from build123d import *

# Parameters (mm, degrees)
F1_DEPTH      = 10
F2_W          = 2
F2_H          = 10
F3_DEPTH      = 13.3
F3_DEPTH_BACK = 11.9
F4_R          = 4.99999


# Not quite as in the source:
# - a fillet or chamfer is up to 0.001 mm smaller than in the source, because OpenCascade refuses the exact size


with BuildPart() as f1:
    # F0 (on Top) → F1 (new body)
    with BuildSketch(Plane.XY):
        with BuildLine():
            Line((-1.25, -5.5), (3.25, -5.5))
            Line((3.25, -5.5), (3.25, 3.499999999))
            ThreePointArc((3.25, 3.499999999), (2.2500000005, 4.499999999), (1.25, 3.5))
            Line((1.25, 3.5), (1.25, -2.5))
            ThreePointArc((1.25, -2.5), (0.9571067812, -3.2071067812), (0.25, -3.5))
            Line((0.25, -3.5), (-0.25, -3.5))
            ThreePointArc((-0.25, -3.5), (-0.9571067812, -3.2071067812), (-1.25, -2.5))
            Line((-1.25, -2.5), (-1.25, 2.5))
            ThreePointArc((-1.25, 2.5), (-0.9571067812, 3.2071067812), (-0.25, 3.5))
            add(Edge.make_bspline(
                [(-1.2744928417, 5.5), (0.3231141309, 5.4264482222), (0.6423479063, 3.9560622536), (-0.25, 3.5)],
                knots=[0, 0, 0, 0, 2.2471282969, 2.2471282969, 2.2471282969, 2.2471282969], degree=3))
            ThreePointArc((-1.2744928417, 5.5), (-2.6728467387, 4.9056773399), (-3.25, 3.5001499804))
            Line((-3.25, 3.5001499804), (-3.25, -3.5))
            ThreePointArc((-3.25, -3.5), (-2.6642135624, -4.9142135624), (-1.25, -5.5))
        make_face()
    extrude(amount=F1_DEPTH)

    # F2 (on Front) → F3 (join, two sides)
    with BuildSketch(Plane.XZ) as f3_sk:
        with Locations((2.25, 5)):
            Rectangle(F2_W, F2_H)
    extrude(amount=F3_DEPTH)
    extrude(f3_sk.sketch, amount=-F3_DEPTH_BACK)

    # F4 (radius 5 in the source; OpenCascade refuses exactly that, so slightly less here)
    f4_edges = [f1.edges().sort_by_distance(p)[0] for p in [
        (2.25, -13.3, 10),
        (2.25, 11.9, 10),
        (2.25, -13.3, 0),
        (2.25, 11.9, 0),
    ]]
    fillet(f4_edges, radius=F4_R)


solid = f1.part
Read the model definition and answer for the solid it produces. Units are mm, in the model's axes. A direction names the side the tool comes from. Coordinates: 2 decimals unless noted, no trailing zeros. Loops run counter-clockwise (first coordinate to the right, second up) from the corner with the lowest first, then second, coordinate; pieces in that order, holes last. Notation, with made-up numbers: (-16.5, 78.5) - (11.5, 78.5) arc R30 ccw to (11.5, 111.5) - close; hole circle Ø3 at (44.25, 73). An arc over 180 degrees is marked (long way). Answer in a Markdown table with one row per item.
Q1. For faces 4 (the flat face through (2, -1, 0)), 5 (the flat face through (0, -5.5, 5)), 6 (the cylindrical face through (-0.949, -3.215, 4.93)), 7 (the flat face through (1.25, 5, 5)), 8 (the cylindrical face through (2.26, -11.8, 8.57)), determine the directions among +Z, -Z, +X, -X, +Y, -Y from which every point of the face is accessible in a straight line to the end or side of a thin tool.
Here are the results:
| item | result |
|---|---|
| face 4 | -Z, +X, -X, +Y, -Y |
| face 5 | +Z, -Z, -X, -Y |
| face 6 | +Z, -Z |
| face 7 | +Z, -Z, +Y |
| face 8 | +Z, +X, -X, -Y |
Q2. Find section C-C on y = -7.5. Write down the section's boundary in (x, z).
Here are the results:
| item | result |
|---|---|
| outline | (1.25, 0) - (3.25, 0) - (3.25, 10) - (1.25, 10) - close |
Q3. Find section D-D on x = -2.5. Write down the section's boundary in (y, z), plus the area to 3 significant figures.
Here are the results:
| item | result |
|---|---|
| outline | (-5.06, 0) - (5.06, 0) - (5.06, 10) - (-5.06, 10) - close |
| area | 101 mm^2 |
Q4. Find section A-A on y = -1. Write down the section's boundary in (x, z).
Here are the results:
| item | result |
|---|---|
| outline | (-3.25, 0) - (-1.25, 0) - (-1.25, 10) - (-3.25, 10) - close; (1.25, 0) - (3.25, 0) - (3.25, 10) - (1.25, 10) - close |
Q5. The mould has two halves that part along X. Classify faces 1 (the flat face through (3.25, -1, 5)), 2 (the cylindrical face through (-0.965, 3.199, 4.93)), 3 (the flat face through (1.25, -9, 5)): pulls with the +X half, pulls with the -X half, needs draft (parallel to the pull), parting line crosses it, or undercut.
Here are the results:
| item | result |
|---|---|
| face 1 | pulls with the +X half |
| face 2 | undercut |
| face 3 | pulls with the -X half |
Q6. Given P1, Ø2.5, axis at y = -11, z = 3.5, coming from the -X side; P2, Ø3, axis at x = -0.5, z = 2, coming from the +Y side; P3, Ø1.2, axis at x = -0.5, z = 3, coming from the -Y side, each flat-ended and moving along its own axis, determine where each tip first touches the part or whether it passes through.
Here are the results:
| item | result |
|---|---|
| P1 | stops at x = 1.25 |
| P2 | stops at y = 5.5 |
| P3 | stops at y = -5.5 |
Q7. Straight lines are drawn through the part: line 1 along X through (y, z) = (2.5, 3); line 2 along X through (y, z) = (-11.25, 6.25); line 3 along Y through (x, z) = (-0.75, 5.25). For each, find the intervals that lie inside material, in ascending order. Write a range as [from, to].
Here are the results:
| item | result |
|---|---|
| line 1 | x = [-3.25, -1.25], [1.25, 3.25] |
| line 2 | x = [1.25, 3.25] |
| line 3 | y = [-5.5, -3.37], [3.37, 5.42] |
